Read the model definition and answer for the solid it produces. Units are mm, in the model's axes. Face numbers are marked on the shaded views. A direction names the side the tool comes from. Coordinates: 2 decimals unless noted, no trailing zeros. Loops run counter-clockwise (first coordinate to the right, second up) from the corner with the lowest first, then second, coordinate; pieces in that order, holes last. Notation, with made-up numbers: M 20,-22 L 54,-22 A18 ccw 54,-12 Z; hole C 76.25,22 d10. An arc over 180 degrees is marked long. One line per item, written item: value. Start each with the question number.
1. Determine the mould class of the marked faces 1, 2 and 3 for opening direction X: +X half, -X half, draft (parallel to the pull), parting line (faces both ways), or undercut.
2. The part is cut by section D-D (x = 19). Write down the section's boundary in (y, z), then the cut area to 3 significant figures.
3. The part is cut by section C-C (y = 12). Write down the section's boundary in (x, z), then the cut area to 3 significant figures.
4. Consider probe 1 along X at (y, z) = (-8, 24.5); probe 2 along X at (y, z) = (17.5, 58.5); probe 3 along Y at (x, z) = (-56, 90). Determine where each line is inside the solid, lowest interval first.
5. Flat-ended cylindrical pins translate along their axes: pin 1 (10 mm diameter, centred on x = -23, z = 64.5, fed in from -Y); pin 2 (14 mm diameter, centred on x = -58.5, z = 60, fed in from -Y); pin 3 (10 mm diameter, centred on x = -21.5, y = 10.5, fed in from +Z). Find the tip coordinate at first contact, or state that the pin passes through.
6. For the marked faces 4, 5 and 6, determine the directions among +Z, -Z, +X, -X, +Y, -Y from which every point of the face is accessible in a straight line to the end or side of a thin tool.
7. The part is cut by section A-A (y = 29.5). Write down the section's boundary in (x, z).
8. The part is cut by section B-B (z = 88.5). Write down the section's boundary in (x, y), then the cut area to 3 significant figures.
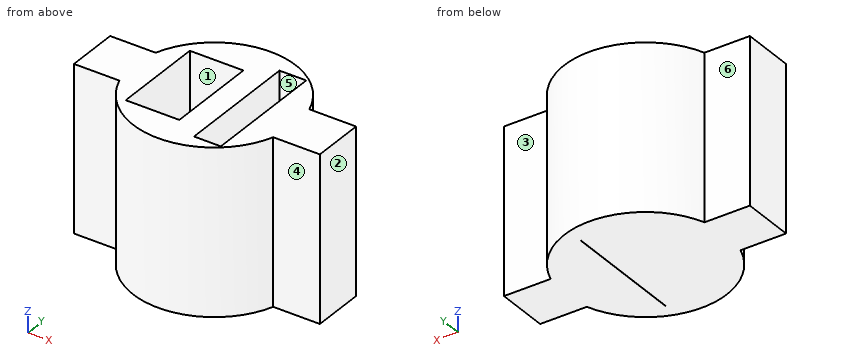
```python
from build123d import *

# Parameters (mm, degrees)
F0_W     = 28.0003916717
F0_H     = 32.2663935487
F0_W_2   = 28.7430296161
F1_DEPTH = 101.6
F2_W     = 34.6587272506
F2_H     = 58.0717623234
F2_W_2   = 16.9384283945
F2_H_2   = 77.3962959647
F3_DEPTH = 12.7


# Not quite as in the source:
# - a feature names something its author has since deleted; it is built from what else it names


with BuildPart() as f1:
    # F0 (on Top) → F1 (new body)
    with BuildSketch(Plane.XY):
        with BuildLine():
            Line((-47.371, 16.1331967744), (-47.371, -16.1331967744))
            ThreePointArc((-47.371, -16.1331967744), (0, -50.0428983889), (47.371, -16.1331967744))
            Line((47.371, -16.1331967744), (47.371, 16.1331967744))
            ThreePointArc((47.371, 16.1331967744), (0, 50.0428983889), (-47.371, 16.1331967744))
        make_face()
        Polygon((-34.1799231236, -29.6225996721), (-34.1799231236, 27.5274003279), (-1.1599231236, 27.5274003279), (-1.1599231236, -29.6225996721), (-8.1120360752, -29.6225996721), align=None, mode=Mode.SUBTRACT)
        Polygon((13.945407662, -38.3726616568), (13.945407662, 37.8273383432), (30.455407662, 37.8273383432), (30.455407662, -38.3726616568), (18.8453282475, -38.3726616568), align=None, mode=Mode.SUBTRACT)
        with Locations((-61.3711958359, 0)):
            Rectangle(F0_W, F0_H)
        with Locations((61.7425148081, 0)):
            Rectangle(F0_W_2, F0_H)
    extrude(amount=F1_DEPTH)

    # F2 (on Top) → F3 (join)
    with BuildSketch(Plane.XY):
        with Locations((-17.2371207664, -0.9217876941)):
            Rectangle(F2_W, F2_H)
        with Locations((22.572400514, -0.1084208488)):
            Rectangle(F2_W_2, F2_H_2)
    extrude(amount=F3_DEPTH)


solid = f1.part
```
Answer block:
1. face 1: undercut
1. face 2: +X half
1. face 3: draft
2. outline: M -46.3,0 L 46.3,0 L 46.3,101.6 L 37.83,101.6 L 37.83,12.7 L -38.37,12.7 L -38.37,101.6 L -46.3,101.6 Z
2. area: 2,630 mm2
3. outline: M -75.37,0 L 13.95,0 L 13.95,101.6 L -1.16,101.6 L -1.16,12.7 L -34.18,12.7 L -34.18,101.6 L -75.37,101.6 Z; M 14.1,0 L 76.11,0 L 76.11,101.6 L 30.46,101.6 L 30.46,12.7 L 14.1,12.7 Z
3. area: 11,000 mm2
4. probe 1: x = -75.37 to -34.18, -1.16 to 13.95, 30.46 to 76.11
4. probe 2: x = -46.88 to -34.18, -1.16 to 13.95, 30.46 to 46.88
4. probe 3: y = -16.13 to 16.13
5. pin 1: stops at y = -46.69
5. pin 2: stops at y = -16.13
5. pin 3: stops at z = 12.7
6. face 4: +Z, -Z, +X, -Y
6. face 5: +Z
6. face 6: +Z, -Z, -X, +Y
7. outline: M -40.42,0 L 13.95,0 L 13.95,101.6 L -40.42,101.6 Z; M 14.1,0 L 40.42,0 L 40.42,101.6 L 30.46,101.6 L 30.46,12.7 L 14.1,12.7 Z
8. outline: M -75.37,-16.13 L -47.37,-16.13 A50.04 ccw 47.37,-16.13 L 76.11,-16.13 L 76.11,16.13 L 47.37,16.13 A50.04 ccw -47.37,16.13 L -75.37,16.13 Z; hole M -34.18,-29.62 L -1.16,-29.62 L -1.16,27.53 L -34.18,27.53 Z; hole M 13.95,-38.37 L 30.46,-38.37 L 30.46,37.83 L 13.95,37.83 Z
8. area: 6,440 mm2
